Source: three-view drawing plus pictorial views. Frame: mm from the lowest corner of the part. A direction names the side the tool comes from. Round coordinates to 2 decimals unless told otherwise and drop trailing zeros. Loops run counter-clockwise (first coordinate to the right, second up) from the corner with the lowest first, then second, coordinate; pieces in that order, holes last. Notation, with made-up numbers: (16, 44) -> (60, 44) arc R24 cw to (60, 68) -> close; hole circle Ø10 at (5.25, 32.5). An arc over 180 degrees is marked (long way). One line per question, with ' | ' between items. Start each with the question number.
Q1. Access query for the marked faces 1, 2 and 3. Directions: +Z, -Z, +X, -X, +Y, -Y. A direction counts if a zero-diameter tool reaches every point of the face in a straight line with its end or side. Return the directions, or none.
Q2. Cut plane A-A on x = 2.8. Return loops of the section in (y, z), and give its area (3 significant figures).
Q3. Contact query for flat-ended pins moving along their axis: P1, Ø1.5, axis at y = 1, z = 10.5, coming from the +X side; P2, Ø1.5, axis at y = 0.5, z = 5.5, coming from the +X side; P3, Ø1.5, axis at x = 1, z = 3.5, coming from the -Y side. Output: stop coordinate, or through.
Q4. Cut plane B-B on y = 2. Return loops of the section in (x, z).
Q5. Cut plane D-D on y = 1.15. Return loops of the section in (x, z), and give its area (3 significant figures).
Q6. Cut plane C-C on z = 8.25. Return loops of the section in (x, y), and give its area (3 significant figures).
Q7. Material intervals for L1, parallel to Z at x = 2.3, y = 1.45; L2, parallel to Z at x = 2, y = 2.65; L3, parallel to Y at x = 2.15, z = 2.5, sorted ascending.
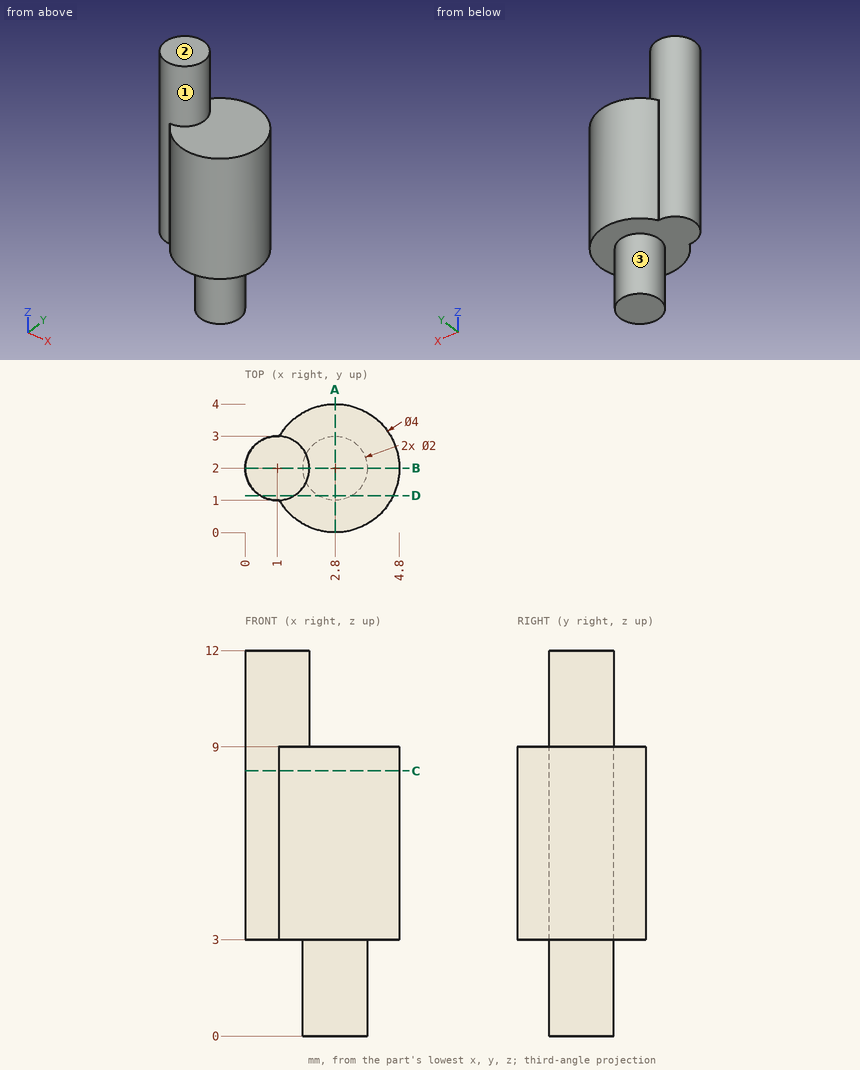
Results:
1) face 1: +Z | face 2: +Z, +X, -X, +Y, -Y | face 3: -Z
2) outline: (0, 3) -> (1, 3) -> (1, 0) -> (3, 0) -> (3, 3) -> (4, 3) -> (4, 9) -> (0, 9) -> close | area: 30.0 mm^2
3) P1: x = 1.97 | P2: x = 4.65 | P3: y = 0.3
4) outline: (0, 3) -> (1.8, 3) -> (1.8, 0) -> (3.8, 0) -> (3.8, 3) -> (4.8, 3) -> (4.8, 9) -> (2, 9) -> (2, 12) -> (0, 12) -> close
5) outline: (0.47, 3) -> (2.27, 3) -> (2.27, 0) -> (3.33, 0) -> (3.33, 3) -> (4.61, 3) -> (4.61, 9) -> (1.53, 9) -> (1.53, 12) -> (0.47, 12) -> close | area: 31.1 mm^2
6) outline: (1, 1) -> (1.07, 1) arc R2 ccw (long way) to (1.07, 3) -> (1, 3) arc R1 ccw to start | area: 13.9 mm^2
7) L1: 0 to 9 | L2: 3 to 9 | L3: 1.24 to 2.76
